Drawing for the job (mm, zero at the part's lowest x, y, z). Round coordinates to 2 decimals unless told otherwise and drop trailing zeros. Loops run counter-clockwise (first coordinate to the right, second up) from the corner with the lowest first, then second, coordinate; pieces in that order, holes last. Notation, with made-up numbers: M 40.25,53 L 47.25,53 A19 cw 47.25,84 Z; hole C 83.25,-22 d11. An arc over 180 degrees is marked long. Put each result on its own line as item: value. Start each with the question number.
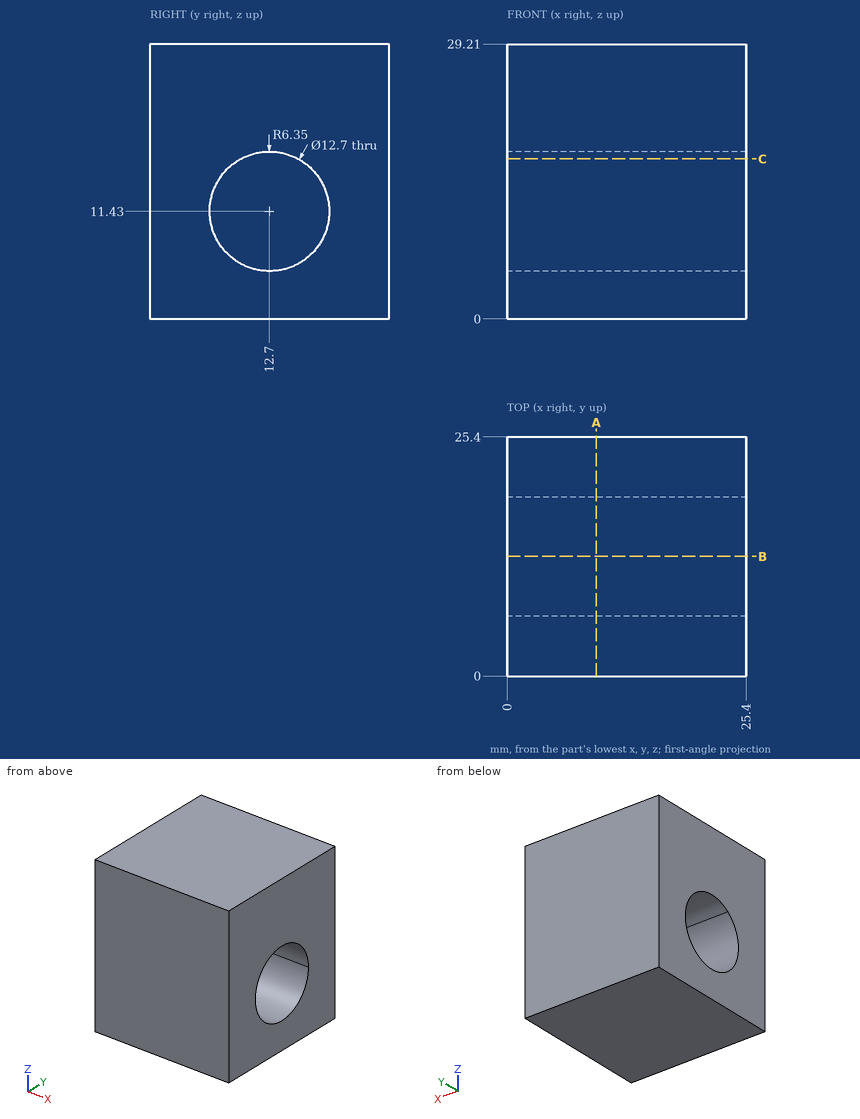
1. Cut at A-A, the plane x = 9.5. Give the cut face in (y, z), and give its area (3 significant figures).
2. Wall check: L1, parallel to Y at x = 19, z = 11.43; L2, parallel to Z at x = 9.25, y = 12.7; L3, parallel to Z at x = 11.5, y = 7. Give the ranges that are in metal, low to high.
3. Cut at B-B, the plane y = 12.7. Give the cut face in (x, z), and give its area (3 significant figures).
4. Cut at C-C, the plane z = 17. Give the cut face in (x, y).
Results list:
1. outline: M 0,0 L 25.4,0 L 25.4,29.21 L 0,29.21 Z; hole M 16.51,16.51 A6.35 ccw long 19.05,11.43 A6.35 ccw Z
1. area: 615 mm^2
2. L1: y = 0 to 6.35, 19.05 to 25.4
2. L2: z = 0 to 5.08, 17.78 to 29.21
2. L3: z = 0 to 8.63, 14.23 to 29.21
3. outline: M 0,0 L 25.4,0 L 25.4,5.08 L 0,5.08 Z; M 0,17.78 L 25.4,17.78 L 25.4,29.21 L 0,29.21 Z
3. area: 419 mm^2
4. outline: M 0,0 L 25.4,0 L 25.4,9.65 L 0,9.65 Z; M 0,15.75 L 25.4,15.75 L 25.4,25.4 L 0,25.4 Z
